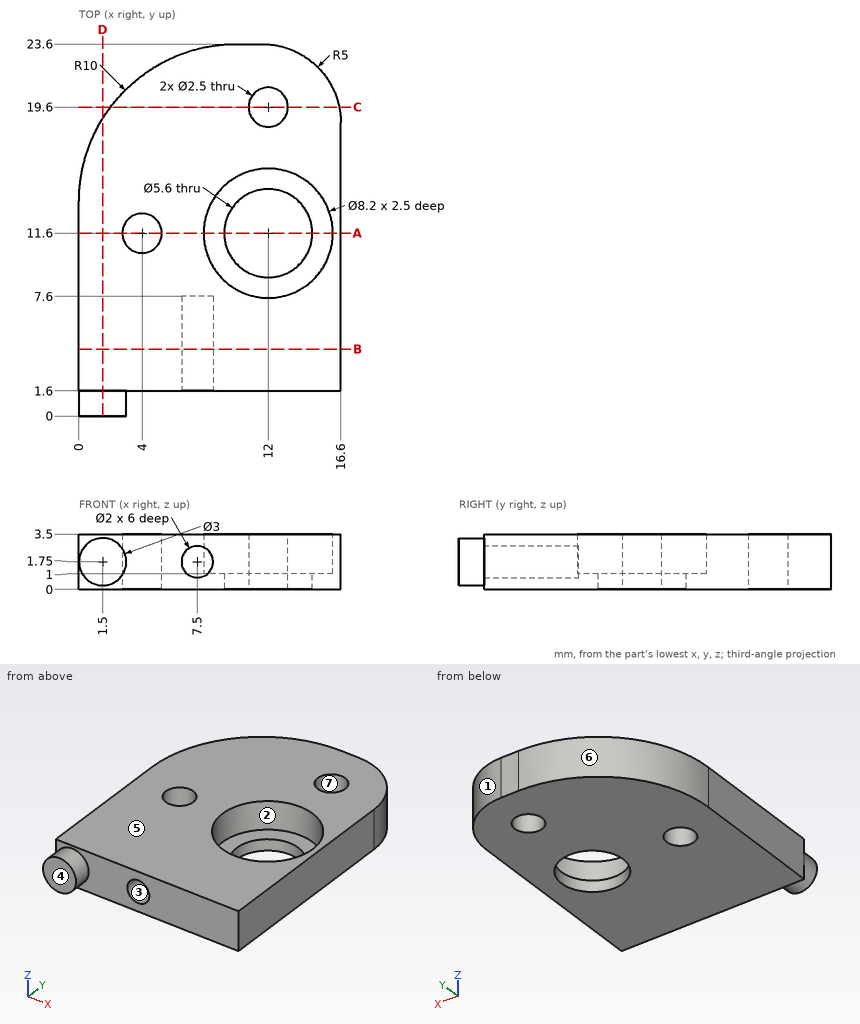
Geometry check sheet. Reference: drawing and pictorial views, mm from the part's lowest x, y, z. A direction names the side the tool comes from. Coordinates: 2 decimals unless noted, no trailing zeros. Write each loop counter-clockwise with the first axis right and the second up, starting at its lowest first coordinate (ties: lowest second). Pieces come first, ordered by that corner, then holes.
Item 1: Access from +Z, -Z, +X, -X, +Y, -Y to the whole of each face (thin tool, end or side, straight path). Record for the marked faces 1, 2 and 3.
Numbers:
face 1: +Z, -Z, +X, +Y
face 2: +Z
face 3: -Y
Item 2: Cross-section at C-C on y = 19.6. Record the boundary of the cut face in (x, z), then the cut area to 3 significant figures.
Numbers:
outline: (2, 0) - (10.75, 0) - (10.75, 3.5) - (2, 3.5) - close; (13.25, 0) - (16.5, 0) - (16.5, 3.5) - (13.25, 3.5) - close
area: 42.0 mm2
Item 3: Mould release check, pull along Y, two halves, no side actions. Record for the marked faces 4, 5, 6 and 7: released by +Y, released by -Y, zero draft, split by the parting line, or undercut.
Numbers:
face 4: released by -Y
face 5: zero draft
face 6: released by +Y
face 7: undercut
Item 4: Cross-section at B-B on y = 4.25. Record the boundary of the cut face in (x, z).
Numbers:
outline: (0, 0) - (16.6, 0) - (16.6, 3.5) - (0, 3.5) - close; hole circle Ø2 at (7.5, 1.75)
Item 5: Cross-section at D-D on x = 1.5. Record the boundary of the cut face in (y, z).
Numbers:
outline: (0, 0.25) - (1.6, 0.25) - (1.6, 0) - (18.87, 0) - (18.87, 3.5) - (1.6, 3.5) - (1.6, 3.25) - (0, 3.25) - close
Item 6: Cross-section at A-A on y = 11.6. Record the boundary of the cut face in (x, z), then the cut area to 4 significant figures.
Numbers:
outline: (0, 0) - (2.75, 0) - (2.75, 3.5) - (0, 3.5) - close; (5.25, 0) - (9.2, 0) - (9.2, 1) - (7.9, 1) - (7.9, 3.5) - (5.25, 3.5) - close; (14.8, 0) - (16.6, 0) - (16.6, 3.5) - (16.1, 3.5) - (16.1, 1) - (14.8, 1) - close
area: 23.25 mm2
Item 7: Depth check by flat-ended pin: pin 1 Ø1 at (x, z) = (7, 1.5) entering from -Y; pin 2 Ø1.2 at (x, z) = (7.5, 1.75) entering from -Y. Enter the tip coordinate at first touch or a pass-through.
Numbers:
pin 1: stops at y = 1.6
pin 2: stops at y = 7.6
Item 8: Scan lines: probe 1 along Y at (x, z) = (12, 0.3); probe 2 along Y at (x, z) = (12, 2.85); probe 3 along X at (y, z) = (10.5, 0.2). Record each from-to range of solid material in increasing order.
Numbers:
probe 1: y = 1.6 to 8.8, 14.4 to 18.35, 20.85 to 23.58
probe 2: y = 1.6 to 7.5, 15.7 to 18.35, 20.85 to 23.58
probe 3: x = 0 to 3.41, 4.59 to 9.43, 14.57 to 16.6
